CAD build for the part. Positions are in the model's coordinates, mm. Face numbers are marked on the shaded views. Round coordinates to 2 decimals unless told otherwise and drop trailing zeros. Loops run counter-clockwise (first coordinate to the right, second up) from the corner with the lowest first, then second, coordinate; pieces in that order, holes last. Notation, with made-up numbers: (85.5, -6) - (112.5, -6) arc R33 cw to (112.5, 26) - close; hole circle Ø10 at (13.25, 20). An arc over 180 degrees is marked (long way). Use one line per item in the form item = value.
from build123d import *

# Parameters (mm, degrees)
SKETCH1_W           = 7.5
SKETCH1_H           = 2.45
BOSS_EXTRUDE1_DEPTH = 5
FILLET1_R           = 0.762
FILLET2_R           = 1.27
CUT_EXTRUDE1_DEPTH  = 4


with BuildPart() as part:
    # Sketch1 → Boss-Extrude1 (new body)
    with BuildSketch(Plane.XY):
        Rectangle(SKETCH1_W, SKETCH1_H)
    extrude(amount=BOSS_EXTRUDE1_DEPTH)

    # Fillet1
    fillet1_edges = [part.edges().sort_by_distance(p)[0] for p in [
        (0, 1.225, 0),
        (-3.75, 1.225, 2.5),
        (3.75, 1.225, 2.5),
    ]]
    fillet(fillet1_edges, radius=FILLET1_R)

    # Fillet2
    fillet2_edges = [part.edges().sort_by_distance(p)[0] for p in [
        (3.75, -1.225, 2.5),
        (-3.75, -1.225, 2.5),
    ]]
    fillet(fillet2_edges, radius=FILLET2_R)

    # Sketch2 → Cut-Extrude1 (cut)
    with BuildSketch(Plane.XY.offset(5)):
        with BuildLine():
            Line((3.496, 0.045), (3.496, 0.463))
            ThreePointArc((3.496, 0.463), (3.347210245, 0.822210245), (2.988, 0.971))
            Line((2.988, 0.971), (-2.988, 0.971))
            ThreePointArc((-2.988, 0.971), (-3.347210245, 0.822210245), (-3.496, 0.463))
            Line((-3.496, 0.463), (-3.496, 0.045))
            ThreePointArc((-3.496, 0.045), (-3.19842049, -0.67342049), (-2.48, -0.971))
            Line((-2.48, -0.971), (2.48, -0.971))
            ThreePointArc((2.48, -0.971), (3.19842049, -0.67342049), (3.496, 0.045))
        make_face()
    extrude(amount=-CUT_EXTRUDE1_DEPTH, mode=Mode.SUBTRACT)


solid = part.part
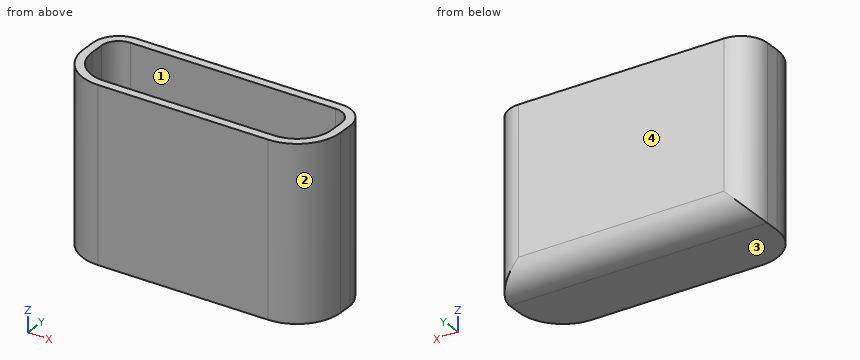
1) Slice it at C-C (y = 0.25). Write the cut outline in (x, z).
Report:
outline = (-3.75, 0) - (3.75, 0) - (3.75, 5) - (3.5, 5) - (3.5, 1) - (-3.5, 1) - (-3.5, 5) - (-3.75, 5) - close
2) Slice it at B-B (x = -1.5). Write the cut outline in (y, z) (3 decimals), plus the area to 3 significant figures.
Report:
outline = (-1.225, 0) - (0.463, 0) arc R0.762 ccw to (1.225, 0.762) - (1.225, 5) - (0.971, 5) - (0.971, 1) - (-0.971, 1) - (-0.971, 5) - (-1.225, 5) - close
area = 4.36 mm^2
3) Slice it at D-D (z = 0.45). Write the cut outline in (x, y) (3 decimals).
Report:
outline = (-3.75, 0.045) arc R1.27 ccw to (-2.48, -1.225) - (2.48, -1.225) arc R1.27 ccw to (3.75, 0.045) - (3.75, 0.463) arc R0.762 ccw to (3.3, 1.158) - (-3.3, 1.158) arc R0.762 ccw to (-3.75, 0.463) - close
4) Slice it at A-A (z = 2.45). Write the cut outline in (x, y) (3 decimals).
Report:
outline = (-3.75, 0.045) arc R1.27 ccw to (-2.48, -1.225) - (2.48, -1.225) arc R1.27 ccw to (3.75, 0.045) - (3.75, 0.463) arc R0.762 ccw to (2.988, 1.225) - (-2.988, 1.225) arc R0.762 ccw to (-3.75, 0.463) - close; hole (-3.496, 0.045) arc R1.016 ccw to (-2.48, -0.971) - (2.48, -0.971) arc R1.016 ccw to (3.496, 0.045) - (3.496, 0.463) arc R0.508 ccw to (2.988, 0.971) - (-2.988, 0.971) arc R0.508 ccw to (-3.496, 0.463) - close
5) Drill centre lines: probe 1 along X at (y, z) = (0.05, 4.5); probe 2 along Y at (x, z) = (1, 2.45) (3 decimals); probe 3 along X at (y, z) = (0.5, 1.4). Where is each one in solid material? Low to high.
Report:
probe_1 = -3.75 to -3.5, 3.5 to 3.75
probe_2 = -1.225 to -0.971, 0.971 to 1.225
probe_3 = -3.75 to -3.49, 3.49 to 3.75
6) Two-plate mould, pull along Y, no slides. Class the marked faces 1, 2, 3 and 4: +Y half, -Y half, draft (parallel to the pull), parting line (faces both ways), or undercut.
Report:
face_1 = undercut
face_2 = -Y half
face_3 = draft
face_4 = +Y half
